Autodesk Inventor part; units mm, degrees
ref_plane "YZ Plane" through (0, 0, 0) normal (1, 0, 0) x (0, 1, 0)
ref_plane "XZ Plane" through (0, 0, 0) normal (0, 1, 0) x (-1, 0, 0)
ref_plane "XY Plane" through (0, 0, 0) normal (0, 0, 1) x (1, 0, 0)
sketch "Sketch1" plane through (0, 0, 0) normal (0, 1, 0) x (-1, 0, 0)
  line L0 (0, 0) -> (-13, 0)
  line L1 (0, 0) -> (-13, 0)
  line L2 (-13, 0) -> (-13, -80)
  line L3 (-13, -80) -> (0, -80)
  line L4 (0, -80) -> (0, 0)
  circle A0 centre (-6.5, -5) radius 1.5
  circle A1 centre (-6.5, -20) radius 1.5
  circle A2 centre (-6.5, -75) radius 1.5
  circle A3 centre (-6.5, -60) radius 1.5
  dimension "d1" = 13
  dimension "d2" = 80
  dimension "d4" = 3
  dimension "d6" = 3
extrude "Extrusion1" add sketch "Sketch1" along normal blind 13
sketch "Sketch2" plane through (13, 0, 0) normal (1, 0, 0) x (0, 0, -1)
  line L0 (0, 13) -> (80, 13)
  line L1 (40, 13) -> (40, 0)
  line L2 (0, 0) -> (80, 0)
  arc A0 (40, 10.2749) -> (40, 2.7251) centre (36, 6.5) ccw
  arc A1 (40, 2.7251) -> (40, 10.2749) centre (44, 6.5) ccw
  dimension "d10" = 11
extrude "Extrusion2" cut sketch "Sketch2" against normal blind 13
sketch "Sketch3" plane through (0, 13, 0) normal (0, 1, 0) x (1, 0, 0)
  line L0 (13, 80) -> (0, 80)
  circle A0 centre (6.5, 75) radius 1.5
  line L1 (13, 0) -> (13, 80)
  point P0 (0, 0)
  point P1 (6.5, 80)
  dimension "d13" = 5
  dimension "d14" = 6.5
properties part number "cella di carico"
Read the model definition and answer for the solid it produces. Units are mm, in the model's axes. Give positions to 0.01 mm unless a question says otherwise; leave off trailing zeros. Loops run counter-clockwise (first coordinate to the right, second up) from the corner with the lowest first, then second, coordinate; pieces in that order, holes last. Notation, with made-up numbers: (6.5, 69.5) -> (51.5, 69.5) arc R17 cw to (51.5, 85.5) -> close; hole circle Ø5 at (-27.5, 5). An arc over 180 degrees is marked (long way). Answer as CSV lines item,"result".
Item 1: Find section C-C on y = 2. Give the vertices of the cut face in (x, z).
Returned:
outline,"(0, -80) -> (13, -80) -> (13, -47.16) -> (0, -47.16) -> close; (0, -40.84) -> (13, -40.84) -> (13, -39.16) -> (0, -39.16) -> close; (0, -32.84) -> (13, -32.84) -> (13, 0) -> (0, 0) -> close; hole circle Ø3 at (6.5, -75); hole circle Ø3 at (6.5, -60); hole circle Ø3 at (6.5, -20); hole circle Ø3 at (6.5, -5)"
Item 2: This flat-tipped pin is pushed along its axis until it touches: pin 1 (1 mm diameter, centred on y = 3, z = -45, fed in from +X). Where does it stop, or does it pass through?
Returned:
pin 1,"passes through"
Item 3: Find section D-D on x = 3.5. Give the vertices of the cut face in (y, z).
Returned:
outline,"(0, -80) -> (13, -80) -> (13, 0) -> (0, 0) -> close; hole (2.73, -40) arc R5.5 ccw (long way) to (10.27, -40) arc R5.5 ccw (long way) to start"
Item 4: Find section B-B on z = -44. Give the vertices of the cut face in (x, y).
Returned:
outline,"(0, 0) -> (13, 0) -> (13, 1) -> (0, 1) -> close; (0, 12) -> (13, 12) -> (13, 13) -> (0, 13) -> close"
Item 5: Find section A-A on y = 6.5. Give the vertices of the cut face in (x, z), plus the area to 3 significant figures.
Returned:
outline,"(0, -80) -> (13, -80) -> (13, -49.5) -> (0, -49.5) -> close; (0, -30.5) -> (13, -30.5) -> (13, 0) -> (0, 0) -> close; hole circle Ø3 at (6.5, -75); hole circle Ø3 at (6.5, -60); hole circle Ø3 at (6.5, -20); hole circle Ø3 at (6.5, -5)"
area,"765 mm²"
Item 6: Consider line 1 (X direction, y = 6.5, z = -75); line 2 (Z direction, x = 6.5, y = 9.75); line 3 (Z direction, x = 6.5, y = 4.75). Determine where each line is inside the solid, lowest interval first. Write a range as [from, to].
Returned:
line 1,"x = [0, 5], [8, 13]"
line 2,"z = [-80, -76.5], [-73.5, -61.5], [-58.5, -48.44], [-31.56, -21.5], [-18.5, -6.5], [-3.5, 0]"
line 3,"z = [-80, -76.5], [-73.5, -61.5], [-58.5, -49.21], [-30.79, -21.5], [-18.5, -6.5], [-3.5, 0]"
Item 7: Determine the mould class of faces 1 (the face through (6, 6, 0)), 2 (the face through (7, 6, -80)), 3 (the face through (6.591, 6.684, -30.503)) for opening direction Z: +Z half, -Z half, draft (parallel to the pull), parting line (faces both ways), or undercut.
Returned:
face 1,"+Z half"
face 2,"-Z half"
face 3,"undercut"
